Part model, mm, in its own coordinate system. A direction names the side the tool comes from. Round coordinates to 2 decimals unless told otherwise and drop trailing zeros. Order: outer loops, then holes, each group sorted by start corner. A loop starts at its lowest first (then second) coordinate and runs counter-clockwise, first axis right, second up. Notation, with made-up numbers: (-25, -31.5) - (8, -31.5) arc R19 cw to (8, -27.5) - close; hole circle Ø10 at (19, 5.5). An arc over 180 degrees is marked (long way). Answer as a JSON object with one key per item and string values.
```python
from build123d import *

# Parameters (mm, degrees)
BOSS_EXTRUDE1_DEPTH = 5
SKETCH2_R           = 2.1
CUT_EXTRUDE1_DEPTH  = 10
BOSS_EXTRUDE2_DEPTH = 5
BOSS_EXTRUDE3_DEPTH = 5
SKETCH5_R           = 2.1
CUT_EXTRUDE2_DEPTH  = 5
BOSS_EXTRUDE4_DEPTH = 5
SKETCH7_W           = 5.4
SKETCH7_H           = 25.4
SKETCH7_H_2         = 5.4
CUT_EXTRUDE4_DEPTH  = 5
SKETCH8_R           = 2.1
SKETCH8_W           = 15.4
SKETCH8_H           = 5.4
SKETCH8_W_2         = 15
SKETCH8_H_2         = 5
SKETCH8_W_3         = 5.4
SKETCH8_H_3         = 15.4
CUT_EXTRUDE5_DEPTH  = 5
SKETCH9_W           = 15
SKETCH9_H           = 5
CUT_EXTRUDE6_DEPTH  = 10
SKETCH10_R          = 2.1
CUT_EXTRUDE7_DEPTH  = 10


with BuildPart() as part:
    # Sketch1 → Boss-Extrude1 (new body)
    with BuildSketch(Plane.XY):
        Polygon((-182, 200), (-182, 180), (-187, 180), (-187, 20), (-182, 20), (-182, 0), (0, 0), (0, 20), (5, 20), (5, 180), (0, 180), (0, 200), align=None)
    extrude(amount=BOSS_EXTRUDE1_DEPTH)

    # Sketch2 → Cut-Extrude1 (cut)
    with BuildSketch(Plane(origin=(0, 0, 0), x_dir=(-1, 0, 0), z_dir=(0, 0, -1))):
        with Locations((-2.5, 139.3)):
            Circle(SKETCH2_R)
        with Locations((-2.5, 37.9)):
            Circle(SKETCH2_R)
        with Locations(Location((184.5, 37.9, 0), (0, 0, 180))):
            Circle(SKETCH2_R)
        with Locations(Location((184.5, 139.3, 0), (0, 0, 180))):
            Circle(SKETCH2_R)
    extrude(amount=-CUT_EXTRUDE1_DEPTH, mode=Mode.SUBTRACT)

    # Sketch3 → Boss-Extrude2 (add)
    with BuildSketch(Plane(origin=(0, 0, 0), x_dir=(-1, 0, 0), z_dir=(0, 0, -1))):
        with BuildLine():
            Line((-5, 136.177501001), (-5, 142.422498999))
            ThreePointArc((-5, 142.422498999), (-6.5, 139.3), (-5, 136.177501001))
        make_face()
    boss_extrude2 = extrude(amount=-BOSS_EXTRUDE2_DEPTH)

    # Sketch4 → Boss-Extrude3 (add)
    with BuildSketch(Plane(origin=(0, 0, 0), x_dir=(-1, 0, 0), z_dir=(0, 0, -1))):
        with BuildLine():
            Line((-5, 34.777501001), (-5, 41.022498999))
            ThreePointArc((-5, 41.022498999), (-6.5, 37.9), (-5, 34.777501001))
        make_face()
    boss_extrude3 = extrude(amount=-BOSS_EXTRUDE3_DEPTH)

    # Mirror1: Boss-Extrude2, Boss-Extrude3 across plane
    add(boss_extrude2.mirror(Plane.ZY.offset(91)))
    add(boss_extrude3.mirror(Plane.ZY.offset(91)))

    # Sketch5 → Cut-Extrude2 (cut)
    with BuildSketch(Plane(origin=(0, 0, 0), x_dir=(-1, 0, 0), z_dir=(0, 0, -1))):
        with Locations((30, 2.5)):
            Circle(SKETCH5_R)
        with Locations((152, 2.5)):
            Circle(SKETCH5_R)
    extrude(amount=-CUT_EXTRUDE2_DEPTH, mode=Mode.SUBTRACT)

    # Sketch6 → Boss-Extrude4 (add)
    with BuildSketch(Plane(origin=(0, 0, 0), x_dir=(-1, 0, 0), z_dir=(0, 0, -1))):
        with BuildLine():
            Line((155.122498999, 0), (148.877501001, 0))
            ThreePointArc((148.877501001, 0), (152, -1.5), (155.122498999, 0))
        make_face()
        with BuildLine():
            Line((33.122498999, 0), (26.877501001, 0))
            ThreePointArc((26.877501001, 0), (30, -1.5), (33.122498999, 0))
        make_face()
    extrude(amount=-BOSS_EXTRUDE4_DEPTH)

    # Sketch7 → Cut-Extrude4 (cut)
    with BuildSketch(Plane.XY.offset(5)):
        with Locations((-30.5, 167.5)):
            Rectangle(SKETCH7_W, SKETCH7_H)
        with Locations((-40.5, 167.5)):
            Rectangle(SKETCH7_W, SKETCH7_H)
        with Locations((-30.5, 132.5)):
            Rectangle(SKETCH7_W, SKETCH7_H_2)
        with Locations((-40.5, 132.5)):
            Rectangle(SKETCH7_W, SKETCH7_H_2)
    cut_extrude4 = extrude(amount=-CUT_EXTRUDE4_DEPTH, mode=Mode.SUBTRACT)

    # Mirror2: Cut-Extrude4 across plane
    add(cut_extrude4.mirror(Plane.ZY.offset(91)), mode=Mode.SUBTRACT)

    # Sketch8 → Cut-Extrude5 (cut)
    # profile 1 of 12: a face of its own
    with BuildSketch(Plane(origin=(0, 0, 0), x_dir=(-1, 0, 0), z_dir=(0, 0, -1))):
        with Locations((90.999998379, 12.5)):
            Circle(SKETCH8_R)
    # profile 2 of 12: a face of its own
    with BuildSketch(Plane(origin=(0, 0, 0), x_dir=(-1, 0, 0), z_dir=(0, 0, -1))):
        with Locations(Location((90.999998379, 187.5, 0), (0, 0, 180))):
            Circle(SKETCH8_R)
    # profile 3 of 12: a face of its own
    with BuildSketch(Plane(origin=(0, 0, 0), x_dir=(-1, 0, 0), z_dir=(0, 0, -1))):
        with Locations((174.499996757, 100)):
            Circle(SKETCH8_R)
    # profile 4 of 12: a face of its own
    with BuildSketch(Plane(origin=(0, 0, 0), x_dir=(-1, 0, 0), z_dir=(0, 0, -1))):
        with Locations(Location((7.5, 100, 0), (0, 0, 180))):
            Circle(SKETCH8_R)
    # profile 5 of 12: a face of its own
    with BuildSketch(Plane(origin=(0, 0, 0), x_dir=(-1, 0, 0), z_dir=(0, 0, -1))):
        with Locations((108.499998379, 187.5)):
            Rectangle(SKETCH8_W, SKETCH8_H)
    # profile 6 of 12: a face of its own
    with BuildSketch(Plane(origin=(0, 0, 0), x_dir=(-1, 0, 0), z_dir=(0, 0, -1))):
        with Locations((73.499998379, 12.5)):
            Rectangle(SKETCH8_W, SKETCH8_H)
        with Locations((73.499998379, 12.5)):
            Rectangle(SKETCH8_W_2, SKETCH8_H_2, mode=Mode.SUBTRACT)
    # profile 7 of 12: a face of its own
    with BuildSketch(Plane(origin=(0, 0, 0), x_dir=(-1, 0, 0), z_dir=(0, 0, -1))):
        with Locations((73.499998379, 187.5)):
            Rectangle(SKETCH8_W, SKETCH8_H)
    # profile 8 of 12: a face of its own
    with BuildSketch(Plane(origin=(0, 0, 0), x_dir=(-1, 0, 0), z_dir=(0, 0, -1))):
        with Locations((108.499998379, 12.5)):
            Rectangle(SKETCH8_W, SKETCH8_H)
    # profile 9 of 12: a face of its own
    with BuildSketch(Plane(origin=(0, 0, 0), x_dir=(-1, 0, 0), z_dir=(0, 0, -1))):
        with Locations((174.499996757, 82.5)):
            Rectangle(SKETCH8_W_3, SKETCH8_H_3)
    # profile 10 of 12: a face of its own
    with BuildSketch(Plane(origin=(0, 0, 0), x_dir=(-1, 0, 0), z_dir=(0, 0, -1))):
        with Locations((174.499996757, 117.5)):
            Rectangle(SKETCH8_W_3, SKETCH8_H_3)
    # profile 11 of 12: a face of its own
    with BuildSketch(Plane(origin=(0, 0, 0), x_dir=(-1, 0, 0), z_dir=(0, 0, -1))):
        with Locations((7.5, 82.5)):
            Rectangle(SKETCH8_W_3, SKETCH8_H_3)
    # profile 12 of 12: a face of its own
    with BuildSketch(Plane(origin=(0, 0, 0), x_dir=(-1, 0, 0), z_dir=(0, 0, -1))):
        with Locations((7.5, 117.5)):
            Rectangle(SKETCH8_W_3, SKETCH8_H_3)
    extrude(amount=-CUT_EXTRUDE5_DEPTH, mode=Mode.SUBTRACT)


with BuildPart() as cut_extrude5_piece_1:
    # of the separate pieces the step leaves, piece 1, a body of its own (cut_extrude5_pieces)
    add(part.part.solids().sort_by_distance((-182, 200, 0))[0])

    # Sketch10 → Cut-Extrude7 (cut)
    with BuildSketch(Plane.XY.offset(5)):
        with BuildLine():
            Line((-148.8, 135.2), (-148.8, 133.208307979))
            ThreePointArc((-148.8, 133.208307979), (-147.314689345, 132.176321717), (-146.193604234, 130.757057274))
            ThreePointArc((-146.193604234, 130.757057274), (-145.216422795, 130.325730949), (-144.2, 129.997385607))
            Line((-144.2, 129.997385607), (-144.2, 135.2))
            Line((-144.2, 135.2), (-138.8, 135.2))
            Line((-138.8, 135.2), (-138.8, 130.013594506))
            ThreePointArc((-138.8, 130.013594506), (-137.394509388, 149.490991099), (-150.702850957, 135.2))
            Line((-150.702850957, 135.2), (-148.8, 135.2))
        make_face()
        Polygon((-149.030035391, 129.647109894), (-149.030035433, 129.8), (-154.030035433, 129.8), (-154.030035391, 129.647108503), align=None)
        with Locations((-141.529997703, 186.747164896)):
            Circle(SKETCH10_R)
        with BuildLine():
            Line((-149.030050697, 184.647109894), (-149.030051718, 188.316347969))
            ThreePointArc((-149.030051718, 188.316347969), (-151.530056924, 188.847109198), (-154.030051718, 188.316298928))
            Line((-154.030051718, 188.316298928), (-154.030050697, 184.647108503))
            Line((-154.030050697, 184.647108503), (-149.030050697, 184.647109894))
        make_face()
    cut_extrude7 = extrude(amount=-CUT_EXTRUDE7_DEPTH, mode=Mode.SUBTRACT)

    # Mirror3: Cut-Extrude7 across plane
    add(cut_extrude7.mirror(Plane(origin=(-91, 0, 0), x_dir=(0, 0, 1), z_dir=(1, 0, 0))), mode=Mode.SUBTRACT)


with BuildPart() as cut_extrude5_piece_2:
    # of the separate pieces the step leaves, piece 2, a body of its own (cut_extrude5_pieces)
    add(part.part.solids().sort_by_distance((-80.999998379, 10, 0))[0])

    # Sketch9 → Cut-Extrude6 (cut)
    with BuildSketch(Plane.XY.offset(5)):
        with Locations((-73.499998379, 12.5)):
            Rectangle(SKETCH9_W, SKETCH9_H)
    extrude(amount=-CUT_EXTRUDE6_DEPTH, mode=Mode.SUBTRACT)


solid = cut_extrude5_piece_1.part
```
Item 1: Tool access for faces 4 (the flat face through (-184, 180, 2)), 5 (the flat face through (-14, 0, 2)), 6 (the flat face through (-92, 0, 2)), 7 (the flat face through (-31, 180.2, 3)): list every direction of +Z, -Z, +X, -X, +Y, -Y with a clear straight run to the whole face (end or side of a thin tool).
Taken from the geometry:
{"face 4": "+Z, -Z, -X, +Y", "face 5": "+Z, -Z, +X, -Y", "face 6": "+Z, -Z, -Y", "face 7": "+Z, -Z"}
Item 2: Drop flat-ended pins along their axis: P1, Ø1.5, axis at x = -138, y = 161.5, coming from the -Z side; P2, Ø2.5, axis at y = 9, z = 1.5, coming from the -X side; P3, Ø1.7, axis at y = 132, z = 2, coming from the +X side. Give the stop position or say it passes through.
Taken from the geometry:
{"P1": "z = 0", "P2": "x = -182", "P3": "x = 5"}
Item 3: Cut at B-B (z = 0.8). State how many separate pieces and enclosed holes the cut face has, plus the area to 3 significant figures.
Taken from the geometry:
{"separate pieces": "1", "enclosed holes": "28", "area": "35,900 mm2"}
Item 4: Two-plate mould, pull along Y, no slides. Class faces 1 (the flat face through (2, 20, 2)), 2 (the flat face through (-90, 200, 2)), 3 (the flat face through (-73, 9.8, 2)): pulls with the +Y half, pulls with the -Y half, needs draft (parallel to the pull), parting line crosses it, or undercut.
Taken from the geometry:
{"face 1": "pulls with the -Y half", "face 2": "pulls with the +Y half", "face 3": "undercut"}
Item 5: Probe L1, parallel to Y at x = -7.5, z = 2.4; L2, parallel to X at y = 78, z = 2.65; L3, parallel to Y at x = -69.5, z = 2. List the from-to ranges inside material, lowest first. Write a range as from..to.
Taken from the geometry:
{"L1": "0..74.8, 90.2..97.9, 102.1..109.8, 125.2..200", "L2": "-187..-177.2, -171.8..-10.2, -4.8..5", "L3": "0..9.8, 15.2..184.8, 190.2..200"}
Item 6: Cut at A-A (y = 49.5). Write the cut outline in (x, z).
Taken from the geometry:
{"outline": "(-187, 0) - (5, 0) - (5, 5) - (-187, 5) - close"}
